Part print with two shaded views. Sizes in mm from the minimum x, y, z corner. Round coordinates to 2 decimals unless told otherwise and drop trailing zeros. Order: outer loops, then holes, each group sorted by start corner. A loop starts at its lowest first (then second) coordinate and runs counter-clockwise, first axis right, second up. Notation, with made-up numbers: (-0.5, 14.25) - (8.5, 14.25) arc R27 cw to (8.5, 44.25) - close; hole circle Ø1 at (-6, 83.25). An arc over 180 degrees is marked (long way). Use one line per item in the form item = value.
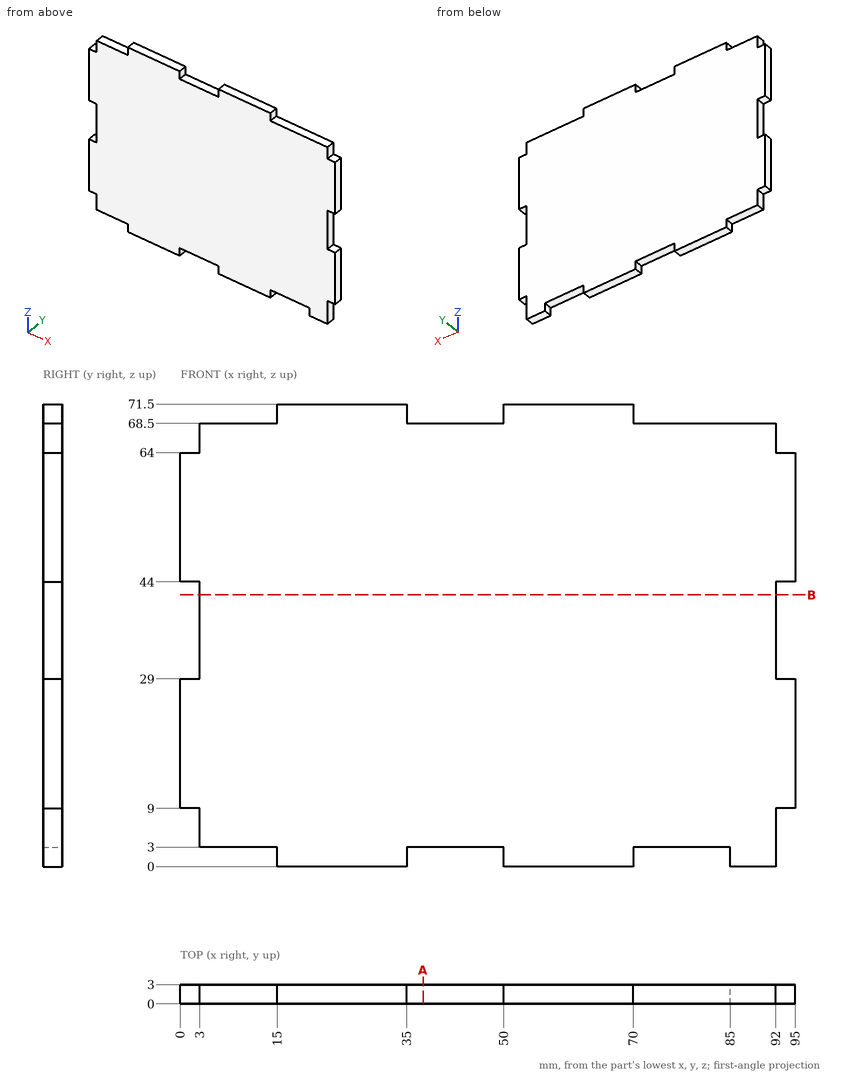
(1) Probe probe 1 along X at (y, z) = (1.7, 37); probe 2 along Z at (x, y) = (6, 2.85); probe 3 along Z at (x, y) = (86, 2.35). List the from-to ranges inside material, lowest first. Write a range as [from, to].
Report:
probe_1 = [3, 92]
probe_2 = [3, 68.5]
probe_3 = [0, 68.5]
(2) Slice it at A-A on x = 37.5. Give the cut face in (y, z), then the cut area to 4 significant figures.
Report:
outline = (0, 3) - (3, 3) - (3, 68.5) - (0, 68.5) - close
area = 196.5 mm2
(3) Pin check, flat tips, straight feed: pin 1 (1.5 mm diameter, centred on y = 2, z = 32.5, fed in from +X); pin 2 (1.5 mm diameter, centred on y = 1.5, z = 69.5, fed in from +X); pin 3 (0.9 mm diameter, centred on x = 94, y = 1, fed in from +Z); pin 4 (3 mm diameter, centred on x = 81.5, z = 29.5, fed in from -Y). Stop position of each tip, or through.
Report:
pin_1 = 92
pin_2 = 70
pin_3 = 64
pin_4 = 0
(4) Slice it at B-B on z = 42. Give the cut face in (x, y).
Report:
outline = (3, 0) - (92, 0) - (92, 3) - (3, 3) - close
